The drawing under review shows one solid part. Ordinate dimensions are in mm from its lowest x, y, z. Coordinates: 2 decimals unless noted, no trailing zeros. Write each loop counter-clockwise with the first axis right and the second up, starting at its lowest first coordinate (ties: lowest second). Pieces come first, ordered by that corner, then holes. Notation, with made-up numbers: (0.5, 50) - (58.5, 50) arc R21 ccw to (58.5, 70) - close; hole circle Ø8 at (-12.75, 74.5). An arc over 180 degrees is marked (long way). Put each result on its own line as item: value. Start each with the question number.
Item 1: Consider section A-A on z = 345. Give the boundary of the cut face in (x, y).
Item 2: For pin 1 (4 mm diameter, centred on y = 16.5, z = 217, fed in from -X); pin 2 (10 mm diameter, centred on x = 9.5, y = 9.5, fed in from +Z) (1 decimal), all flat-tipped, find the tip position at first contact; note any pin that passes through.
Item 3: Consider section B-B on x = 7. Give the boundary of the cut face in (y, z) (1 decimal), then the cut area to 3 significant figures.
Item 4: To check wall thickness, follow L1, parallel to X at y = 8.25, z = 361.5; L2, parallel to Z at x = 5, y = 10.75; L3, parallel to Z at x = 14.75, y = 8.75 (1 decimal). State the ranges of each line that lie inside material, in increasing order. Write a range as [from, to].
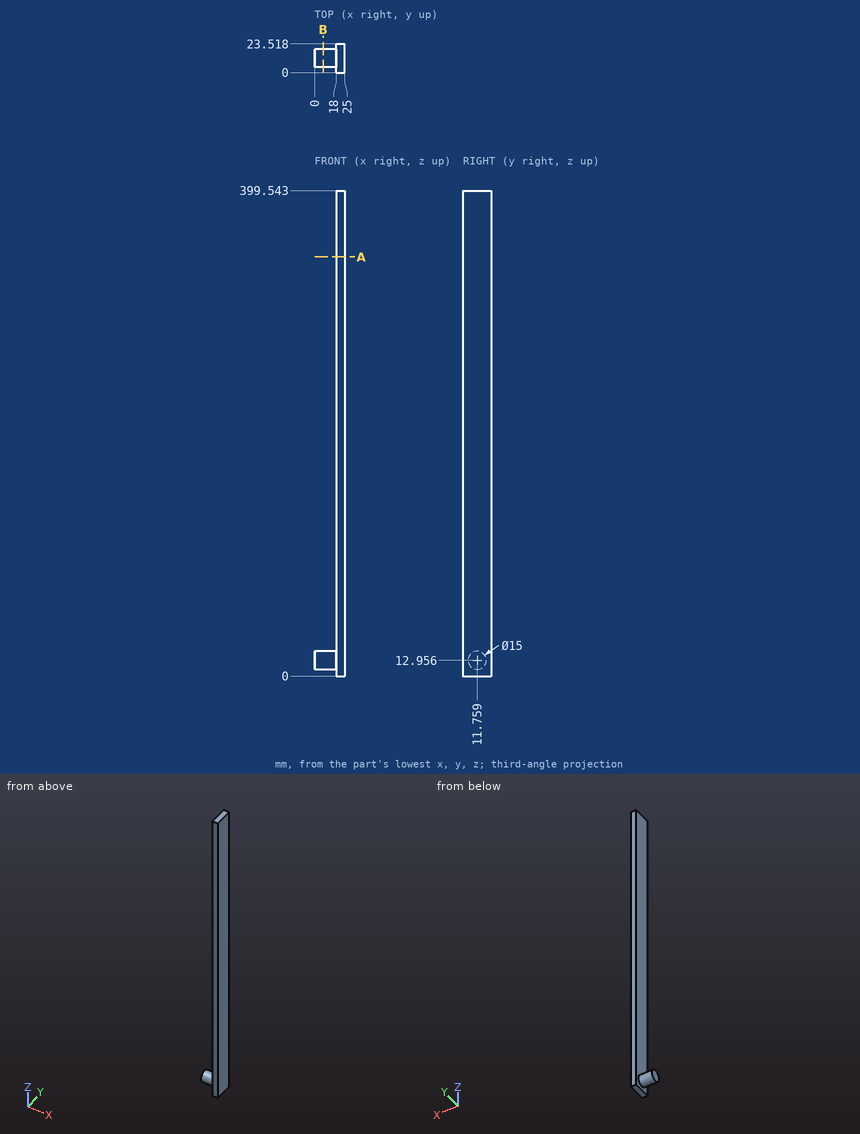
Report:
1. outline: (18, 0) - (25, 0) - (25, 23.52) - (18, 23.52) - close
2. pin 1: x = 18
2. pin 2: z = 20.5
3. outline: circle Ø15 at (11.8, 13)
3. area: 177 mm²
4. L1: [18, 25]
4. L2: [5.52, 20.39]
4. L3: [6.1, 19.8]
